Part model, mm, in its own coordinate system. Face numbers are marked on the shaded views. A direction names the side the tool comes from. Round coordinates to 2 decimals unless told otherwise and drop trailing zeros. Write each loop counter-clockwise with the first axis right and the second up, starting at its lowest first coordinate (ties: lowest second). Pieces come first, ordered by that corner, then holes. Notation, with made-up numbers: (32.5, 17) -> (91.5, 17) arc R14 cw to (91.5, 40) -> close; hole circle Ø1 at (44.25, 53.5). An arc over 180 degrees is marked (long way). Return JSON: item names as keys, results as strings. Group by question number.
(1) Saw through at A-A (x = -7.5). List the corners of the cut face in (y, z), plus the area to 3 significant figures.
(2) Saw through at C-C (z = 6). State how many separate pieces and enclosed holes the cut face has, plus the area to 3 significant figures.
(3) Tool access for the marked faces 1, 2 and 3: list every direction of +Z, -Z, +X, -X, +Y, -Y with a clear straight run to the whole face (end or side of a thin tool).
(4) Drill centre lines: L1, parallel to Z at x = -37, y = 0; L2, parallel to X at y = 0.5, z = 10; L3, parallel to Z at x = -7, y = 0. Where is each one in solid material? Low to high. Write a range as from..to.
(5) Saw through at B-B (z = 30.5). List the corners of the cut face in (x, y).
(6) Mould opens along X. For the marked faces 4, 5 and 6 say: +X half, -X half, draft (parallel to the pull), parting line (faces both ways), or undercut.
(7) Drop flat-ended pins along their axis: pin 1 Ø4 at (x, z) = (-23.5, -13.5) entering from -Y; pin 2 Ø5 at (x, z) = (-6.5, -7) entering from -Y; pin 3 Ø7.5 at (y, z) = (14.5, -14) entering from +X. Give the stop position or say it passes through.
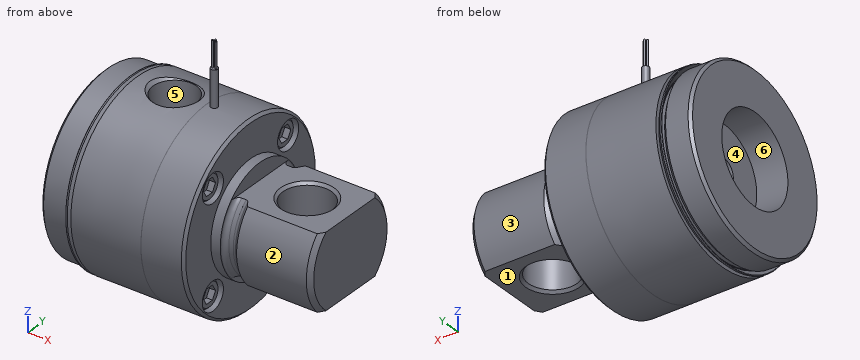
from build123d import *

# Parameters (mm, degrees)
HOLE1_D              = 8.4328
HOLE1_DEPTH          = 5.08
LPATTERN1_COUNT      = 2
LPATTERN1_PITCH      = 29.994055444
LPATTERN1_COUNT_DIR2 = 2
LPATTERN1_PITCH_DIR2 = 29.994055444
LPATTERN2_COUNT      = 2
LPATTERN2_PITCH      = 29.994055444
LPATTERN2_COUNT_DIR2 = 2
LPATTERN2_PITCH_DIR2 = 29.994055444
CUT_EXTRUDE1_DEPTH   = 1.778
LPATTERN3_COUNT      = 2
LPATTERN3_PITCH      = 29.994055444
LPATTERN3_COUNT_DIR2 = 2
LPATTERN3_PITCH_DIR2 = 29.994055444
SKETCH10_W           = 1.016
SKETCH10_H           = 13.2715
SKETCH11_W           = 0.254
SKETCH11_H           = 7.583714286
SKETCH12_W           = 0.254
SKETCH12_H           = 7.583714286
SKETCH13_W           = 7.583714286
SKETCH13_H           = 0.254
SKETCH17_W           = 53.086
SKETCH17_H           = 106.172
SKETCH17_W_2         = 21.844
SKETCH17_H_2         = 53.086
CUT_EXTRUDE2_DEPTH   = 29.464


with BuildPart() as part:
    # Sketch1 → Revolve1 (revolve)
    with BuildSketch(Plane.XY):
        Polygon((-42.8752, 0), (-42.8752, 24.8158), (-42.1132, 25.5778), (-35.4838, 25.5778), (-34.417, 24.511), (-33.3502, 24.511), (-33.3502, 26.543), (-12.7127, 26.5303), (-12.6746, 26.543), (-0.762, 26.543), (0, 25.781), (0, 0), align=None)
    revolve(axis=Axis((0, 0, 0), (-1, 0, 0)))

    # Sketch2 → Revolve2 (revolve)
    with BuildSketch(Plane.XY):
        with BuildLine():
            Line((-34.93160107, 26.318757951), (-32.800553898, 24.18771078))
            Line((-32.800553898, 24.18771078), (-32.477264678, 24.511))
            Line((-32.477264678, 24.511), (-34.458464678, 26.4922))
            Line((-34.458464678, 26.4922), (-34.859759021, 26.4922))
            ThreePointArc((-34.859759021, 26.4922), (-34.953625181, 26.429480637), (-34.93160107, 26.318757951))
        make_face()
    revolve(axis=Axis((-34.458464678, 0, 0), (-1, 0, 0)))

    # Hole1
    with Locations(Plane(origin=(0, 0, 0), x_dir=(0, 0, -1), z_dir=(1, 0, 0))):
        with Locations((-14.997027722, 14.997027722)):
            hole1 = Hole(HOLE1_D / 2, depth=HOLE1_DEPTH)

    # LPattern1: Hole1 2 × 2
    with Locations(*[(0, -j * LPATTERN1_PITCH_DIR2, -i * LPATTERN1_PITCH) for i in range(LPATTERN1_COUNT) for j in range(LPATTERN1_COUNT_DIR2) if (i, j) != (0, 0)]):
        add(hole1, mode=Mode.SUBTRACT)

    # Sketch6 → Revolve3 (revolve)
    with BuildSketch(Plane(origin=(0, 0, 0), x_dir=(1, 0, 0), z_dir=(0, -0.707106781, 0.707106781))):
        Polygon((-5.08, 21.209), (-5.08, 25.00376), (-1.397, 25.00376), (-1.016, 24.62276), (-1.016, 21.209), align=None)
    revolve3 = revolve(axis=Axis((-1.016, 14.997027722, 14.997027722), (-1, 0, 0)))

    # LPattern2: Revolve3 2 × 2
    with Locations(*[(0, -j * LPATTERN2_PITCH_DIR2, -i * LPATTERN2_PITCH) for i in range(LPATTERN2_COUNT) for j in range(LPATTERN2_COUNT_DIR2) if (i, j) != (0, 0)]):
        add(revolve3)

    # Sketch8 → Cut-Extrude1 (cut)
    with BuildSketch(Plane(origin=(-1.016, 0, 0), x_dir=(0, 0, -1), z_dir=(1, 0, 0))):
        Polygon((-17.105227722, 16.21419756), (-17.105227722, 13.779857885), (-14.997027722, 12.562688047), (-12.888827722, 13.779857885), (-12.888827722, 16.21419756), (-14.997027722, 17.431367397), align=None)
    cut_extrude1 = extrude(amount=-CUT_EXTRUDE1_DEPTH, mode=Mode.SUBTRACT)

    # LPattern3: Cut-Extrude1 2 × 2
    with Locations(*[(0, -j * LPATTERN3_PITCH_DIR2, -i * LPATTERN3_PITCH) for i in range(LPATTERN3_COUNT) for j in range(LPATTERN3_COUNT_DIR2) if (i, j) != (0, 0)]):
        add(cut_extrude1, mode=Mode.SUBTRACT)

    # Sketch10 → Revolve4 (revolve)
    with BuildSketch(Plane(origin=(0, 0, 0), x_dir=(1, 0, 0), z_dir=(0, 1, 0))):
        with Locations((-10.16, -30.52445)):
            Rectangle(SKETCH10_W, SKETCH10_H)
    revolve(axis=Axis((-10.668, 0, 37.1602), (0, 0, -1)))

    # Sketch11 → Revolve5 (revolve)
    with BuildSketch(Plane(origin=(0, 0, 0), x_dir=(1, 0, 0), z_dir=(0, 1, 0))):
        with Locations((-11.049, -40.952057143)):
            Rectangle(SKETCH11_W, SKETCH11_H)
    revolve(axis=Axis((-11.176, 0, 44.743914286), (0, 0, -1)))

    # Sketch12 → Revolve6 (revolve)
    with BuildSketch(Plane(origin=(0, 0, 0), x_dir=(1, 0, 0), z_dir=(0, 1, 0))):
        with Locations((-10.033, -40.952057143)):
            Rectangle(SKETCH12_W, SKETCH12_H)
    revolve(axis=Axis((-10.16, 0, 44.743914286), (0, 0, -1)))

    # Sketch13 → Revolve7 (revolve)
    with BuildSketch(Plane(origin=(-10.668, 0, 0), x_dir=(0, 0, -1), z_dir=(1, 0, 0))):
        with Locations((-40.952057143, 0.635)):
            Rectangle(SKETCH13_W, SKETCH13_H)
    revolve(axis=Axis((-10.668, 0.508, 37.1602), (0, 0, 1)))

    # Sketch14 → Cut-Revolve1 (revolve, cut)
    with BuildSketch(Plane.XY):
        Polygon((-42.8752, 0), (-42.8752, 13.1699), (-33.7058, 13.1699), (-33.7058, 3.81), (-12.7, 3.81), (-12.7, 12.7), (-5.08, 12.7), (-5.08, 0), align=None)
    revolve(axis=Axis((-5.08, 0, 0), (-1, 0, 0)), mode=Mode.SUBTRACT)

    # Sketch15 → Cut-Revolve2 (revolve, cut)
    with BuildSketch(Plane(origin=(0, 0, 0), x_dir=(1, 0, 0), z_dir=(0, 1, 0))):
        Polygon((-22.352, 0), (-16.671585745, -3.279588699), (-16.671585745, -3.429), (-15.979865896, -25.585630358), (-15.022496254, -26.543), (-22.352, -26.543), align=None)
    revolve(axis=Axis((-22.352, 0, 26.543), (0, 0, -1)), mode=Mode.SUBTRACT)

    # Sketch16 → Revolve8 (revolve)
    with BuildSketch(Plane.XY):
        with BuildLine():
            Line((0, 0), (0, 15.84325))
            Line((0, 15.84325), (2.794, 15.84325))
            Line((2.794, 15.84325), (2.794, 15.6337))
            ThreePointArc((2.794, 15.6337), (3.195732339, 14.663832339), (4.1656, 14.2621))
            Line((4.1656, 14.2621), (5.477064678, 14.2621))
            ThreePointArc((5.477064678, 14.2621), (6.001953274, 14.366506833), (6.446932339, 14.663832339))
            Line((6.446932339, 14.663832339), (7.6581, 15.875))
            Line((7.6581, 15.875), (28.20416, 15.875))
            Line((28.20416, 15.875), (29.464, 14.61516))
            Line((29.464, 14.61516), (29.464, 0))
            Line((29.464, 0), (0, 0))
        make_face()
    revolve(axis=Axis((29.464, 0, 0), (-1, 0, 0)))

    # Sketch17 → Cut-Extrude2 (cut)
    with BuildSketch(Plane(origin=(2.794, 0, 0), x_dir=(0, 0, -1), z_dir=(1, 0, 0))):
        Rectangle(SKETCH17_W, SKETCH17_H)
        Rectangle(SKETCH17_W_2, SKETCH17_H_2, mode=Mode.SUBTRACT)
    extrude(amount=CUT_EXTRUDE2_DEPTH, mode=Mode.SUBTRACT)

    # Sketch18 → Cut-Revolve3 (revolve, cut)
    with BuildSketch(Plane(origin=(0, 0, 0), x_dir=(1, 0, 0), z_dir=(0, 1, 0))):
        Polygon((16.764, 10.922), (24.7015, 10.922), (23.9395, 10.16), (23.9395, -10.16), (24.7015, -10.922), (16.764, -10.922), align=None)
    revolve(axis=Axis((16.764, 0, 10.922), (0, 0, -1)), mode=Mode.SUBTRACT)


solid = part.part
Computed values:
{
 "1": {"outline": "circle Ø53.09 at (0, 0); hole circle Ø25.4 at (0, 0)", "area": "1,710 mm2"},
 "2": {"separate pieces": "1", "enclosed holes": "3", "area": "2,390 mm2"},
 "3": {"face 1": "-Z, +X, +Y, -Y", "face 2": "+X, -Y", "face 3": "+X, +Y"},
 "4": {"L1": "-25.58..-13.17, 13.17..25.58", "L2": "-33.71..-28.22, -16.49..-12.7, -5.08..9.61, 23.92..29.46", "L3": "-26.54..-12.7, 12.7..26.54"},
 "5": {"outline": "circle Ø2.03 at (-10.67, 0)"},
 "6": {"face 4": "-X half", "face 5": "undercut", "face 6": "draft"},
 "7": {"pin 1": "y = -23.92", "pin 2": "y = -26.16", "pin 3": "x = 0"}
}
